```python
from build123d import *

# Parameters (mm, degrees)
BLANKSKE_W                 = 100
BLANKSKE_H                 = 12.75
BLANK_DEPTH                = 20
TOOTHCUTSIM_DEPTH          = 103.77432802
TEETHCUTS_COUNT            = 22
TEETHCUTS_PITCH            = 4.712388975
SALIENTE_EXTRUIR1_DEPTH    = 10
CORTAR_EXTRUIR1_DEPTH      = 103.77432802
CORTAR_EXTRUIR1_DEPTH_BACK = 0.25
CROQUIS12_W                = 30
CROQUIS12_H                = 10.100558753
CROQUIS13_W                = 99.75
CROQUIS13_H                = 14.5
SALIENTE_EXTRUIR6_DEPTH    = 13
CROQUIS14_R                = 7.25
CROQUIS14_R_2              = 3.4
SALIENTE_EXTRUIR7_DEPTH    = 3
CROQUIS15_R                = 3.4
SALIENTE_EXTRUIR8_DEPTH    = 30
CORTAR_EXTRUIR2_DEPTH      = 111.878875355
CORTAR_EXTRUIR2_DEPTH_BACK = 111.878875355
CROQUIS16_W                = 6.2
CROQUIS16_H                = 3.2


with BuildPart() as part:
    # BlankSke → Blank (new body)
    with BuildSketch(Plane.XY):
        with Locations((50, 6.375)):
            Rectangle(BLANKSKE_W, BLANKSKE_H)
    extrude(amount=-BLANK_DEPTH)

    # TooCutSkeSim → ToothCutSim (cut, through all)
    with BuildSketch(Plane.XY):
        Polygon((0.852189273, 9.375), (-0.852189273, 9.375), (-1.731592507, 12.7754), (1.731592507, 12.7754), align=None)
    toothcutsim = extrude(amount=-TOOTHCUTSIM_DEPTH, mode=Mode.SUBTRACT)

    # TeethCuts: ToothCutSim ×22
    with Locations(*[(i * TEETHCUTS_PITCH, 0, 0) for i in range(1, TEETHCUTS_COUNT)]):
        add(toothcutsim, mode=Mode.SUBTRACT)

    # Croquis1 → Saliente-Extruir1 (add)
    with BuildSketch(Plane.XY):
        Polygon((99.812357748, 9.375), (98.107979202, 9.375), (97.235144855, 12.75), (95.97280312, 12.75), (95.099968773, 9.375), (93.395590227, 9.375), (92.52275588, 12.75), (91.260414145, 12.75), (90.387579798, 9.375), (88.683201252, 9.375), (87.810366905, 12.75), (86.54802517, 12.75), (85.675190823, 9.375), (83.970812277, 9.375), (83.09797793, 12.75), (81.835636195, 12.75), (80.962801848, 9.375), (79.258423302, 9.375), (78.385588955, 12.75), (77.12324722, 12.75), (76.250412873, 9.375), (74.546034327, 9.375), (73.67319998, 12.75), (72.410858245, 12.75), (71.538023898, 9.375), (69.833645352, 9.375), (68.960811005, 12.75), (67.69846927, 12.75), (66.825634923, 9.375), (65.121256377, 9.375), (64.24842203, 12.75), (62.986080295, 12.75), (62.113245948, 9.375), (60.408867402, 9.375), (59.536033055, 12.75), (58.27369132, 12.75), (57.400856973, 9.375), (55.696478427, 9.375), (54.82364408, 12.75), (53.561302345, 12.75), (52.688467998, 9.375), (50.984089452, 9.375), (50.111255105, 12.75), (48.84891337, 12.75), (47.976079023, 9.375), (46.271700477, 9.375), (45.39886613, 12.75), (44.136524395, 12.75), (43.263690048, 9.375), (41.559311502, 9.375), (40.686477155, 12.75), (39.42413542, 12.75), (38.551301073, 9.375), (36.846922527, 9.375), (35.97408818, 12.75), (34.711746445, 12.75), (33.838912098, 9.375), (32.134533552, 9.375), (31.261699205, 12.75), (29.99935747, 12.75), (29.126523123, 9.375), (27.422144577, 9.375), (26.54931023, 12.75), (25.286968495, 12.75), (24.414134148, 9.375), (22.709755602, 9.375), (21.836921255, 12.75), (20.57457952, 12.75), (19.701745173, 9.375), (17.997366627, 9.375), (17.12453228, 12.75), (15.862190545, 12.75), (14.989356198, 9.375), (13.284977652, 9.375), (12.412143305, 12.75), (11.14980157, 12.75), (10.276967223, 9.375), (8.572588677, 9.375), (7.69975433, 12.75), (6.437412595, 12.75), (5.564578248, 9.375), (3.860199702, 9.375), (2.987365355, 12.75), (1.72502362, 12.75), (0.852189273, 9.375), (0, 9.375), (0, 0), (100, 0), (100, 10.100558753), align=None)
    extrude(amount=SALIENTE_EXTRUIR1_DEPTH)

    # Croquis12 → Cortar-Extruir1 (cut, two sides: drawn at the far end of the back side and taken through both)
    with BuildSketch(Plane(origin=(100, 0, 0), x_dir=(0, 0, -1), z_dir=(1, 0, 0)).offset(-CORTAR_EXTRUIR1_DEPTH_BACK)):
        with Locations((5, 5.050279377)):
            Rectangle(CROQUIS12_W, CROQUIS12_H)
    extrude(amount=CORTAR_EXTRUIR1_DEPTH + CORTAR_EXTRUIR1_DEPTH_BACK, mode=Mode.SUBTRACT)

    # Croquis13 → Saliente-Extruir6 (add)
    with BuildSketch(Plane.XZ):
        with Locations((49.875, -5)):
            Rectangle(CROQUIS13_W, CROQUIS13_H)
    extrude(amount=SALIENTE_EXTRUIR6_DEPTH)

    # Croquis14 → Saliente-Extruir7 (add)
    # profile 1 of 2: a face of its own
    with BuildSketch(Plane.XZ.offset(13)):
        with Locations(Location((14, -5, 0), (0, 0, 270))):
            Circle(CROQUIS14_R)
        with Locations(Location((14, -5, 0), (0, 0, 270))):
            Circle(CROQUIS14_R_2, mode=Mode.SUBTRACT)
    # profile 2 of 2: a face of its own
    with BuildSketch(Plane.XZ.offset(13)):
        with Locations(Location((87.8, -5, 0), (0, 0, 270))):
            Circle(CROQUIS14_R)
        with Locations(Location((87.8, -5, 0), (0, 0, 270))):
            Circle(CROQUIS14_R_2, mode=Mode.SUBTRACT)
    extrude(amount=SALIENTE_EXTRUIR7_DEPTH)

    # Croquis15 → Saliente-Extruir8 (add)
    with BuildSketch(Plane.XZ.offset(13)):
        with Locations(Location((87.8, -5, 0), (0, 0, 270))):
            Circle(CROQUIS15_R)
        with Locations(Location((14, -5, 0), (0, 0, 270))):
            Circle(CROQUIS15_R)
    extrude(amount=SALIENTE_EXTRUIR8_DEPTH)

    # Croquis16 → Cortar-Extruir2 (cut, two sides: drawn at the far end of the back side and taken through both)
    with BuildSketch(Plane.XY.offset(2.25).offset(-CORTAR_EXTRUIR2_DEPTH_BACK)):
        with Locations((43.1, -5.5)):
            Rectangle(CROQUIS16_W, CROQUIS16_H)
        with Locations((31.1, -5.5)):
            Rectangle(CROQUIS16_W, CROQUIS16_H)
        with Locations((55.1, -5.5)):
            Rectangle(CROQUIS16_W, CROQUIS16_H)
        with Locations((67.1, -5.5)):
            Rectangle(CROQUIS16_W, CROQUIS16_H)
        with Locations((79.1, -5.5)):
            Rectangle(CROQUIS16_W, CROQUIS16_H)
        with Locations((91.1, -5.5)):
            Rectangle(CROQUIS16_W, CROQUIS16_H)
    extrude(amount=CORTAR_EXTRUIR2_DEPTH + CORTAR_EXTRUIR2_DEPTH_BACK, mode=Mode.SUBTRACT)


solid = part.part
```
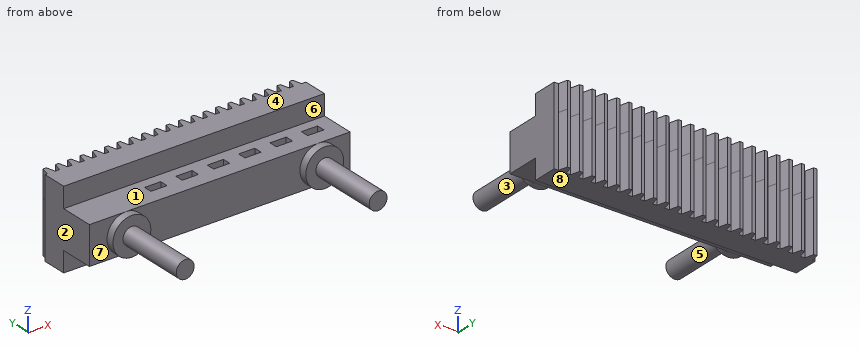
The model under review builds one solid part; all positions refer to its coordinate system, in mm. Face numbers are marked on the shaded views. A direction names the side the tool comes from. Round coordinates to 2 decimals unless told otherwise and drop trailing zeros. Order: outer loops, then holes, each group sorted by start corner. A loop starts at its lowest first (then second) coordinate and runs counter-clockwise, first axis right, second up. Notation, with made-up numbers: (9.5, 84.5) - (68.5, 84.5) arc R21 ccw to (68.5, 91.5) - close; hole circle Ø6 at (23.25, 71.5). An arc over 180 degrees is marked (long way). Answer in a Markdown table with one row per item.
(1) Take a section at C-C on y = -1. Write out the cut boundary in (x, z).
Result set:
| item | result |
|---|---|
| outline | (0, -12.25) - (99.75, -12.25) - (99.75, 2.25) - (0, 2.25) - close |
(2) Take a section at B-B on z = -5. Count the separate pieces of the cut face and the enclosed holes in it, plus the area to 3 significant figures.
Result set:
| item | result |
|---|---|
| separate pieces | 1 |
| enclosed holes | 6 |
| area | 2,720 mm2 |
(3) Take a section at A-A on y = -38. Write out the cut boundary in (x, z).
Result set:
| item | result |
|---|---|
| outline | circle Ø6.8 at (14, -5); circle Ø6.8 at (87.8, -5) |
(4) Mouldability with a two-part tool opening along X and no side actions: class the marked faces 1, 2 and 3 as released by +X, released by -X, zero draft, split by the parting line, or undercut.
Result set:
| item | result |
|---|---|
| face 1 | zero draft |
| face 2 | released by -X |
| face 3 | undercut |
(5) Machinability: for the marked faces 4, 5, 6, 7 and 8, which of the approach directions +Z, -Z, +X, -X, +Y, -Y give a long, thin tool a straight path to every point of the face, cutting with its end or side? Answer none if there is none.
Result set:
| item | result |
|---|---|
| face 4 | +Z, +X, -X, +Y, -Y |
| face 5 | -Y |
| face 6 | +Z, +X, -X, -Y |
| face 7 | -X, -Y |
| face 8 | -Z, +X, -X, +Y, -Y |
(6) Clearance check with flat-ended pins moving along their axes: P1, Ø4, axis at y = -36.5, z = -0.5, coming from the -X side; P2, Ø6.5, axis at x = 73, y = -9.5, coming from the +Z side; P3, Ø12, axis at x = 64, y = -16.5, coming from the -Z side. State where each tip first meets the part, or that it passes through.
Result set:
| item | result |
|---|---|
| P1 | stops at x = 11.7 |
| P2 | stops at z = 2.25 |
| P3 | stops at z = -12.25 |
(7) For line 1 (Y direction, x = 40, z = 4.25); line 2 (Y direction, x = 42.5, z = 4.75) (3 decimals); line 3 (X direction, y = -37, z = -5.5), list the stretches that pass through material, from the lowest coordinate up. Write a range as from..to.
Result set:
| item | result |
|---|---|
| line 1 | y = 0..12.75 |
| line 2 | y = 0..9.375 |
| line 3 | x = 10.64..17.36, 84.44..91.16 |
